Could you check a few things on this drawing? It's one solid part, dimensions in mm from its lowest x, y, z. A direction names the side the tool comes from. Coordinates: 2 decimals unless noted, no trailing zeros. Order: outer loops, then holes, each group sorted by start corner. A loop starts at its lowest first (then second) coordinate and runs counter-clockwise, first axis right, second up.
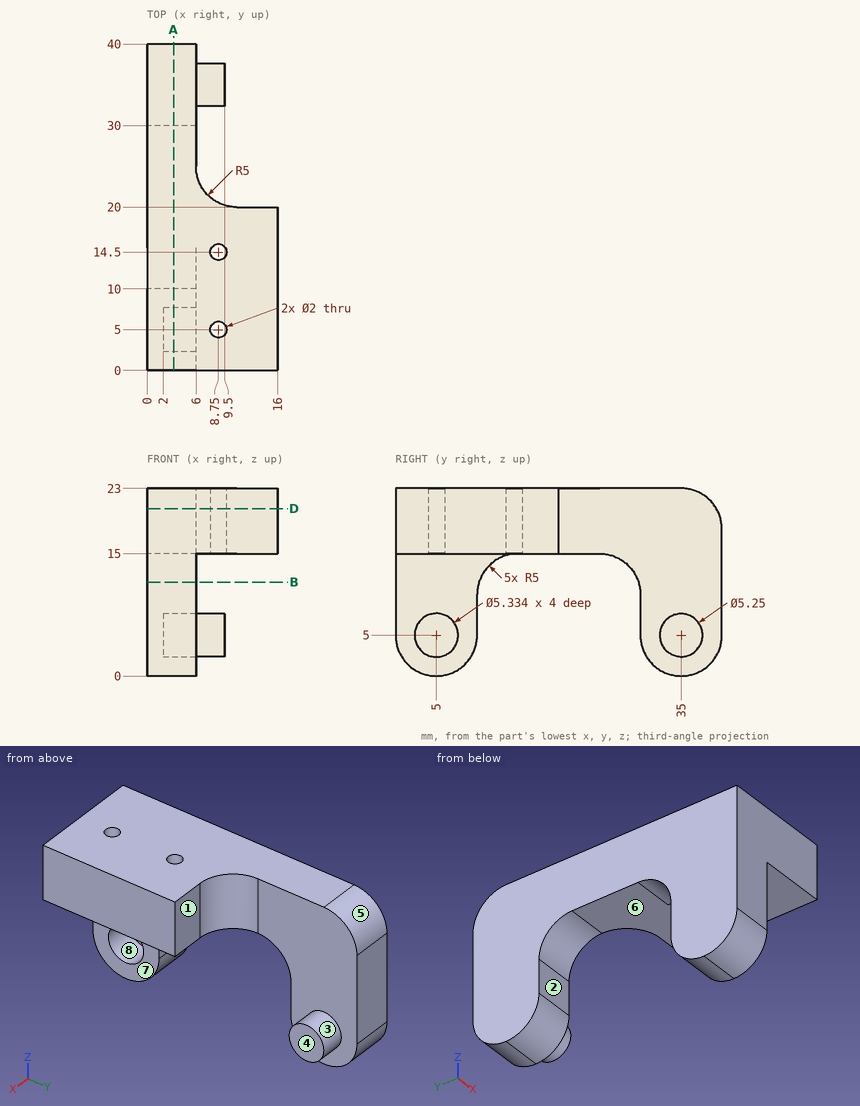
1. I'm going to push flat-ended pins straight in: pin 1 (2.5 mm diameter, centred on y = 6, z = 5.5, fed in from +X); pin 2 (1 mm diameter, centred on y = 28, z = 18.5, fed in from +X); pin 3 (1.5 mm diameter, centred on x = 14, z = 20.5, fed in from +Y). Where does each tip first touch, or does it pass through?
Completed:
pin 1: stops at x = 2
pin 2: stops at x = 6
pin 3: stops at y = 20
2. Imagine slicing it at B-B on z = 11.5. Please give me the cut outline in (x, y).
Completed:
outline: (0, 0) - (6, 0) - (6, 10.23) - (0, 10.23) - close; (0, 29.77) - (6, 29.77) - (6, 40) - (0, 40) - close
3. Please list where these lines run through material, in increasing order: probe 1 along Y at (x, z) = (8.75, 19); probe 2 along X at (y, z) = (14.5, 17.5); probe 3 along X at (y, z) = (35, 10.5).
Completed:
probe 1: y = 0 to 4, 6 to 13.5, 15.5 to 20.53
probe 2: x = 0 to 7.75, 9.75 to 16
probe 3: x = 0 to 6
4. Thinking about a two-plate mould opening in Y: for the marked faces 5, 6, 7 and 8, which applies, pulls with the +Y half, pulls with the -Y half, needs draft (parallel to the pull), parting line crosses it, or undercut?
Completed:
face 5: pulls with the +Y half
face 6: undercut
face 7: needs draft
face 8: undercut
5. Imagine slicing it at D-D on z = 20.5. Please give me the cut outline in (x, y).
Completed:
outline: (0, 0) - (16, 0) - (16, 20) - (11, 20) arc R5 cw to (6, 25) - (6, 39.33) - (0, 39.33) - close; hole circle Ø2 at (8.75, 5); hole circle Ø2 at (8.75, 14.5)
6. Imagine slicing it at A-A on x = 3.25. Please give me the cut outline in (y, z).
Completed:
outline: (0, 5) arc R5 ccw to (10, 5) - (10, 10) arc R5 cw to (15, 15) - (25, 15) arc R5 cw to (30, 10) - (30, 5) arc R5 ccw to (40, 5) - (40, 18) arc R5 ccw to (35, 23) - (0, 23) - close; hole circle Ø5.33 at (5, 5)
7. On a 3-axis mill with a long thin cutter (end or side, diameter ignored), from which of +Z, -Z, +X, -X, +Y, -Y can I reach the whole of each face in a straight line? I mean the marked faces 1, 2, 3 and 4. Say none if no direction works.
Completed:
face 1: +Z, -Z, +X, +Y
face 2: -Z, +X, -X
face 3: +X
face 4: +Z, -Z, +X, +Y, -Y
